Check sheet for the modelled part. Datum: model origin and axes. Units: mm. A direction names the side the tool comes from. Coordinates: 2 decimals unless noted, no trailing zeros. Loops run counter-clockwise (first coordinate to the right, second up) from the corner with the lowest first, then second, coordinate; pieces in that order, holes last.
```python
from build123d import *

# Parameters (mm, degrees)
SKIZZE7_W                            = 4.8
SKIZZE7_H                            = 4.8
AUFSATZ_LINEAR_AUSTRAGEN3_DEPTH      = 5
SKIZZE7_3_W                          = 15
SKIZZE7_3_H                          = 15
SKIZZE7_3_W_2                        = 4.8
SKIZZE7_3_H_2                        = 4.8
AUFSATZ_LINEAR_AUSTRAGEN4_DEPTH      = 5
AUFSATZ_LINEAR_START                 = -38
SKIZZE7_4_W                          = 15
SKIZZE7_4_H                          = 15
AUFSATZ_LINEAR_AUSTRAGEN5_DEPTH      = 5
AUFSATZ_LINEAR_AUSTRAGEN6_DEPTH      = 15
SCHNITT_LINEAR_AUSTRAGEN6_REACH      = 50.07
SCHNITT_LINEAR_AUSTRAGEN7_REACH      = 49.357
SCHNITT_LINEAR_AUSTRAGEN7_END_RADIUS = 21.470910554
SKIZZE12_W                           = 26
SKIZZE12_H                           = 11


with BuildPart() as part:
    # Skizze7 (on Front Plane) → Aufsatz-Linear austragen3 (new body)
    with BuildSketch(Plane.XY):
        with Locations((2.4, -2.4)):
            Rectangle(SKIZZE7_W, SKIZZE7_H)
    extrude(amount=AUFSATZ_LINEAR_AUSTRAGEN3_DEPTH)

    # Skizze7<3> (on Front Plane) → Aufsatz-Linear austragen4 (add)
    with BuildSketch(Plane.XY):
        with Locations((-0.1, -2.4)):
            Rectangle(SKIZZE7_3_W, SKIZZE7_3_H)
        with Locations((2.4, -2.4)):
            Rectangle(SKIZZE7_3_W_2, SKIZZE7_3_H_2, mode=Mode.SUBTRACT)
        with Locations((2.4, -2.4)):
            Rectangle(SKIZZE7_3_W_2, SKIZZE7_3_H_2)
    extrude(amount=-AUFSATZ_LINEAR_AUSTRAGEN4_DEPTH)



with BuildPart() as body_2:
    # Skizze7<4> → Aufsatz-Linear austragen5 (new body)
    with BuildSketch(Plane.XY.offset(AUFSATZ_LINEAR_START)):
        with Locations((-0.1, -2.4)):
            Rectangle(SKIZZE7_4_W, SKIZZE7_4_H)
    extrude(amount=AUFSATZ_LINEAR_AUSTRAGEN5_DEPTH)


with BuildPart() as part_1:
    add(part.part)

    add(body_2.part)  # Aufsatz-Linear austragen6 merges body 2
    # Skizze9 → Aufsatz-Linear austragen6 (add)
    with BuildSketch(Plane(origin=(0, 5.1, 0), x_dir=(1, 0, 0), z_dir=(0, 1, 0))):
        with BuildLine():
            Line((-7.6, 0), (-7.6, 5))
            ThreePointArc((-7.6, 5), (-14.804650534, 19), (-7.6, 33))
            Line((-7.6, 33), (-7.6, 38))
            ThreePointArc((-7.6, 38), (-19.070910554, 19), (-7.6, 0))
        make_face()
    extrude(amount=-AUFSATZ_LINEAR_AUSTRAGEN6_DEPTH)

    # Skizze11 → Schnitt-Linear austragen6 (cut, up to next)
    with BuildSketch(Plane(origin=(0, 0, -38), x_dir=(-1, 0, 0), z_dir=(0, 0, -1)), mode=Mode.PRIVATE) as schnitt_linear_austragen6_sk1:
        with BuildLine():
            Line((-3.9, -0.337840937), (-3.9, -4.462159063))
            ThreePointArc((-3.9, -4.462159063), (-1.242956353, -4.672388611), (0.15, -2.4))
            ThreePointArc((0.15, -2.4), (-1.242956353, -0.127611389), (-3.9, -0.337840937))
        make_face()
    schnitt_linear_austragen6_tool1 = extrude(schnitt_linear_austragen6_sk1.sketch, amount=-SCHNITT_LINEAR_AUSTRAGEN6_REACH, mode=Mode.PRIVATE) & part_1.part
    add(schnitt_linear_austragen6_tool1.solids().sort_by_distance((2.063945, -2.4, -38))[0], mode=Mode.SUBTRACT)

    # Schnitt-Linear austragen7: up to this cylinder (the profile starts inside it)
    schnitt_linear_austragen7_end = Plane(origin=(2.4, -2.4, -19), z_dir=(0, 1, 0)) * Cylinder(SCHNITT_LINEAR_AUSTRAGEN7_END_RADIUS, 142.655821107, mode=Mode.PRIVATE)
    # Skizze12 → Schnitt-Linear austragen7 (cut, up to the surface)
    with BuildSketch(Plane(origin=(7.4, 0, 0), x_dir=(0, 0, -1), z_dir=(1, 0, 0)), mode=Mode.PRIVATE) as schnitt_linear_austragen7_sk1:
        with Locations((19, -2.4)):
            Rectangle(SKIZZE12_W, SKIZZE12_H)
    schnitt_linear_austragen7_tool1 = extrude(schnitt_linear_austragen7_sk1.sketch, amount=-SCHNITT_LINEAR_AUSTRAGEN7_REACH, mode=Mode.PRIVATE) & schnitt_linear_austragen7_end
    add(schnitt_linear_austragen7_tool1.solids().sort_by_distance((7.4, -2.4, -19))[0], mode=Mode.SUBTRACT)


solid = part_1.part
```
1) Depth check by flat-ended pin: pin 1 (8 mm diameter, centred on x = -14, z = -20.5, fed in from +Y); pin 2 (3 mm diameter, centred on y = -8.5, z = -12.5, fed in from -X); pin 3 (3 mm diameter, centred on x = -13, y = -4, fed in from -Z); pin 4 (6 mm diameter, centred on y = -1, z = 0.5, fed in from -X). Enter the tip coordinate at first touch or a pass-through.
Answer sheet:
pin 1: stops at y = 5.1
pin 2: stops at x = -18.48
pin 3: stops at z = -35.36
pin 4: stops at x = -11.34
2) Scan lines: line 1 (Z direction, x = -6, y = -0.5); line 2 (Y direction, x = -11.5, z = -30); line 3 (Z direction, x = -10.75, y = -1.5). Record each from-to range of solid material in increasing order.
Answer sheet:
line 1: z = -38 to -33, -5 to 0
line 2: y = -9.9 to -7.9, 3.1 to 5.1
line 3: z = -35.97 to -32, -6 to -2.03
3) Section check B-B on y = -6.5. Enter the section's corners in (x, z).
Answer sheet:
outline: (-14.69, -32) arc R21.47 ccw to (-7.6, -38) - (7.4, -38) - (7.4, -33) - (-7.6, -33) arc R17.2 cw to (-8.87, -32) - close; (-14.69, -6) - (-8.87, -6) arc R17.2 cw to (-7.6, -5) - (7.4, -5) - (7.4, 0) - (-7.6, 0) arc R21.47 ccw to start
4) Section check D-D on x = 0.5. Enter the section's corners in (y, z).
Answer sheet:
outline: (-9.9, -38) - (-4.1, -38) - (-4.1, -33) - (-9.9, -33) - close; (-9.9, -5) - (5.1, -5) - (5.1, 0) - (0, 0) - (0, 5) - (-4.8, 5) - (-4.8, 0) - (-9.9, 0) - close; (-0.7, -38) - (5.1, -38) - (5.1, -33) - (-0.7, -33) - close
5) Section check C-C on z = -27. Enter the section's corners in (x, y).
Answer sheet:
outline: (-17.52, -9.9) - (-12.83, -9.9) - (-12.83, -7.9) - (-17.52, -7.9) - close; (-17.52, 3.1) - (-12.83, 3.1) - (-12.83, 5.1) - (-17.52, 5.1) - close
6) Section check A-A on x = -17. Enter the section's corners in (y, z), plus the area to 3 significant figures.
Answer sheet:
outline: (-9.9, -28.2) - (-7.9, -28.2) - (-7.9, -9.8) - (-9.9, -9.8) - close; (3.1, -28.2) - (5.1, -28.2) - (5.1, -9.8) - (3.1, -9.8) - close
area: 73.6 mm2
7) Mould release check, pull along Y, two halves, no side actions. Record for faces 1 (the flat face through (3.9, -2, -36)), 2 (the flat face through (-12, -2, -32)), 3 (the flat face through (4.8, -2, 2)), 4 (the flat face through (2, -4.8, 2)): +Y half, -Y half, draft (parallel to the pull), parting line (faces both ways), or undercut.
Answer sheet:
face 1: undercut
face 2: undercut
face 3: draft
face 4: -Y half
8) Set-up check for faces 5 (the flat face through (0, -2, 2)), 6 (the flat face through (-15, 3.1, -19)), 7 (the flat face through (0, -2, -5)): record each of +Z, -Z, +X, -X, +Y, -Y from which the full face is reachable in a straight line by a thin tool's end or side.
Answer sheet:
face 5: +Z, -X, +Y, -Y
face 6: +X, -X
face 7: +X, +Y, -Y
